Autodesk Inventor part; units mm, degrees
ref_plane "YZ Plane" through (0, 0, 0) normal (1, 0, 0) x (0, 1, 0)
ref_plane "XZ Plane" through (0, 0, 0) normal (0, 1, 0) x (-1, 0, 0)
ref_plane "XY Plane" through (0, 0, 0) normal (0, 0, 1) x (1, 0, 0)
sketch "スケッチ1" plane through (0, 0, 0) normal (0, 1, 0) x (-1, 0, 0)
  circle A0 centre (0, 0) radius 39.25
  dimension "d0" = 78.5
extrude "押し出し1" add sketch "スケッチ1" along normal blind 32
sketch "スケッチ2" plane through (0, 32, 0) normal (0, 1, 0) x (1, 0, 0)
  circle A0 centre (0, 0) radius 32.65
  dimension "d3" = 65.3
extrude "押し出し2" cut sketch "スケッチ2" against normal blind 13.5
sketch "スケッチ3" plane through (0, 32, 0) normal (0, 1, 0) x (1, 0, 0)
  circle A0 centre (0, 0) radius 36.5
  point P0 (-36.5, 0)
  point P1 (-27.9606, -23.4617)
  point P2 (-6.3382, -35.9455)
  point P3 (18.25, -31.6099)
  point P4 (34.2988, -12.4837)
  point P5 (34.2988, 12.4837)
  point P6 (18.25, 31.6099)
  point P7 (-6.3382, 35.9455)
  point P8 (-27.9606, 23.4617)
  dimension "d6" = 73
  dimension "d9" = 360
hole "穴1" at (-36.5, 32, 0) at (-27.9606, 32, 23.4617) at (-6.3382, 32, 35.9455) at (18.25, 32, 31.6099) at (34.2988, 32, 12.4837) at (34.2988, 32, -12.4837) at (18.25, 32, -31.6099) at (-6.3382, 32, -35.9455) at (-27.9606, 32, -23.4617) direction (0, -1, 0) diameter 3.4 end through all
sketch "スケッチ4" plane through (0, 32, 0) normal (0, 1, 0) x (1, 0, 0)
  circle A0 centre (0, 0) radius 39.25
  line L0 (38.3222, -8.4837) -> (-38.3222, -8.4837)
  line L1 (0, 0) -> (39.25, 0)
  circle A1 centre (34.2988, -12.4837) radius 1.7
  line L2 (38.3222, 8.4837) -> (-38.3222, 8.4837)
  dimension "d18" = 4
extrude "押し出し3" cut sketch "スケッチ4" against normal blind 13.5 contours A0 L0 L2
sketch "スケッチ5" plane through (0, 18.5, 0) normal (0, 1, 0) x (1, 0, 0)
  circle A0 centre (-36.5, 0) radius 1.7
  circle A1 centre (-36.5, 0) radius 3
  point P0 (0, 0)
  dimension "d21" = 6
extrude "押し出し4" [suppressed]
sketch "スケッチ6" plane through (0, 0, 0) normal (0, -1, 0) x (1, 0, 0)
  circle A0 centre (0, 0) radius 15
  dimension "d24" = 30
extrude "押し出し5" add sketch "スケッチ6" along normal blind 4
sketch "スケッチ7" plane through (0, -4, 0) normal (0, -1, 0) x (1, 0, 0)
  circle A0 centre (0, 0) radius 6
  dimension "d27" = 12
extrude "押し出し6" cut sketch "スケッチ7" against normal blind 40
sketch "スケッチ8" plane through (0, -4, 0) normal (0, -1, 0) x (1, 0, 0)
  circle A0 centre (0, 0) radius 6
  circle A1 centre (0, 0) radius 11
  dimension "d30" = 22
extrude "押し出し7" cut sketch "スケッチ8" against normal blind 5
properties part number "servofixpart_forR2"
Work out the finished part from the listing and answer in its coordinate system (mm). A direction names the side the tool comes from. Round coordinates to 2 decimals unless told otherwise and drop trailing zeros. Order: outer loops, then holes, each group sorted by start corner. A loop starts at its lowest first (then second) coordinate and runs counter-clockwise, first axis right, second up. Notation, with made-up numbers: M 28.5,82 L 67.5,82 A26 ccw 67.5,112 Z; hole C -33,86.25 d6. An arc over 180 degrees is marked long. One line per item, written item: value.
Q1. Find section D-D on x = 18.25. Write down the section's boundary in (y, z).
Derived:
outline: M 0,-34.75 L 32,-34.75 L 32,-33.31 L 0,-33.31 Z; M 0,-29.91 L 32,-29.91 L 32,-27.07 L 18.5,-27.07 L 18.5,27.07 L 32,27.07 L 32,29.91 L 0,29.91 Z; M 0,33.31 L 32,33.31 L 32,34.75 L 0,34.75 Z
Q2. Find section B-B on z = 0. Write down the section's boundary in (x, y), then the cut area to 3 significant figures.
Derived:
outline: M -39.25,0 L -38.2,0 L -38.2,18.5 L -39.25,18.5 Z; M -34.8,0 L -15,0 L -15,-4 L -11,-4 L -11,1 L -6,1 L -6,18.5 L -34.8,18.5 Z; M 6,1 L 11,1 L 11,-4 L 15,-4 L 15,0 L 39.25,0 L 39.25,18.5 L 6,18.5 Z
area: 1,190 mm²
Q3. Determine the mould class of faces 1 (the face through (-17, 0, 1)), 2 (the face through (18.18, 15.78, 29.91)), 3 (the face through (-37.438, 15.776, -11.79)) for opening direction Z: released by +Z, released by -Z, zero draft, split by the parting line, or undercut.
Derived:
face 1: zero draft
face 2: undercut
face 3: split by the parting line
Q4. Find section A-A on x = 0. Write down the section's boundary in (y, z), then the cut area to 3 significant figures.
Derived:
outline: M -4,-15 L 0,-15 L 0,-39.25 L 32,-39.25 L 32,-32.65 L 18.5,-32.65 L 18.5,-6 L 1,-6 L 1,-11 L -4,-11 Z; M -4,11 L 1,11 L 1,6 L 18.5,6 L 18.5,32.65 L 32,32.65 L 32,39.25 L 0,39.25 L 0,15 L -4,15 Z
area: 1,430 mm²
Q5. Straight lines are drawn through the part: line 1 (Z direction, x = 34, y = 12.5); line 2 (Z direction, x = 18, y = 6); line 3 (X direction, y = 10.5, z = -0.5). For each, find the intervals that lie inside material, in ascending order.
Derived:
line 1: -19.61 to -14.16, -10.81 to 10.81, 14.16 to 19.61
line 2: -34.88 to -33.29, -29.93 to 29.93, 33.29 to 34.88
line 3: -39.25 to -38.12, -34.88 to -5.98, 5.98 to 39.25
Q6. Find section C-C on y = 5. Give the number of separate pieces and of enclosed holes in the cut face, then the cut area to 4 significant figures.
Derived:
separate pieces: 1
enclosed holes: 10
area: 4,645 mm²
Q7. Flat-ended cylindrical pins translate along their axes: pin 1 (11 mm diameter, centred on x = 1, z = 2.5, fed in from -Y); pin 2 (3.5 mm diameter, centred on x = -35, y = 25.5, fed in from +Z); pin 3 (12 mm diameter, centred on y = 20, z = 17.5, fed in from -X); pin 4 (2 mm diameter, centred on x = -6.34, z = -35.95, fed in from +Y). Find the tip coordinate at first contact, or state that the pin passes through.
Derived:
pin 1: y = 1
pin 2: z = 20.86
pin 3: x = -37.53
pin 4: through
Q8. For faces 4 (the face through (5, 1, -5)), 5 (the face through (35, 25, -8.484)), 6 (the face through (-0.598, 25.344, 32.645)), determine the directions among +Z, -Z, +X, -X, +Y, -Y from which every point of the face is accessible in a straight line to the end or side of a thin tool.
Derived:
face 4: -Y
face 5: +X, -X, +Y
face 6: +Y
